Here's how the part is built. I have some questions about the finished solid (model axes, mm). A direction names the side the tool comes from. Coordinates: 2 decimals unless noted, no trailing zeros. Write each loop counter-clockwise with the first axis right and the second up, starting at its lowest first coordinate (ties: lowest second). Pieces come first, ordered by that corner, then holes.
Item 1: I want a section at A-A (y = -18.4). Please give me the cut outline in (x, z).
Item 2: For faces 1 (the face through (2.75, -8, -3)), 2 (the face through (4, -15, 4)), 3 (the face through (3, -7.8, 0)), 4 (the face through (5.25, -15, 0)), 5 (the face through (-3.25, 17, 0)), which set-ups out of +Z, -Z, +X, -X, +Y, -Y let a thin tool reach every point of the face, with its end or its side?
Item 3: If we mould it in two halves opening along Y, with no side actions, what happens to faces 6 (the face through (3, -19, -2.75)), 7 (the face through (4, -15, -4)), 8 (the face through (0, 25, 4)), 9 (the face through (4.757, -15.822, 0.338))? For each: pulls with the +Y half, pulls with the -Y half, needs draft (parallel to the pull), parting line crosses it, or undercut.
Item 4: I want a section at D-D (y = -24). Please give me the cut outline in (x, z).
Item 5: Please list where these lines run through material, in increasing order: line 1 (Y direction, x = -7, z = -4.25); line 2 (Y direction, x = 4.9, z = 0); line 3 (Y direction, x = 0.5, z = 0.25).
Item 6: I'm going to push flat-ended pins straight in: P1, Ø1.5, axis at y = 10.5, z = 2, coming from the -X side; P2, Ø4, axis at x = -6, z = 0.5, coming from the +Y side; P3, Ø0.8, axis at x = 4.5, y = -12.5, coming from the -Z side; P4, Ø4, axis at y = -14.5, z = -6.5, coming from the +X side. Where does each tip first touch, or does it pass through?
Item 7: I want a section at B-B (z = 0). Please give me the cut outline in (x, y), and give its area (3 significant figures).
Item 8: I want a section at C-C (x = 0). Please give me the cut outline in (y, z), and give its area (3 significant figures).
from build123d import *

# Parameters (mm, degrees)
SKETCH3_R           = 10
BOSS_EXTRUDE1_DEPTH = 25
SKETCH4_W           = 2.5
SKETCH4_H           = 8
BOSS_EXTRUDE2_DEPTH = 30
CUT_EXTRUDE1_REACH  = 37.108
SKETCH5_R           = 2.6
SKETCH6_W           = 5.5
SKETCH6_H           = 21.2
CUT_EXTRUDE2_DEPTH  = 1.5
SKETCH7_W           = 17
SKETCH7_H           = 7
CUT_EXTRUDE3_DEPTH  = 6
SKETCH8_W           = 2
SKETCH8_H           = 7
CUT_EXTRUDE4_DEPTH  = 4


with BuildPart() as part:
    # Sketch3 → Boss-Extrude1 (new body)
    with BuildSketch(Plane(origin=(0, 0, 0), x_dir=(1, 0, 0), z_dir=(0, 1, 0))):
        with Locations(Location((0, 0, 0), (0, 0, 270))):
            Circle(SKETCH3_R)
    extrude(amount=BOSS_EXTRUDE1_DEPTH)

    # Sketch4 → Boss-Extrude2 (add)
    with BuildSketch(Plane(origin=(0, 0, 0), x_dir=(-1, 0, 0), z_dir=(0, -1, 0))):
        with Locations((-4, 0)):
            Rectangle(SKETCH4_W, SKETCH4_H)
    extrude(amount=BOSS_EXTRUDE2_DEPTH)

    # Sketch5 → Cut-Extrude1 (cut, up to next)
    with BuildSketch(Plane(origin=(5.25, 0, 0), x_dir=(0, 0, -1), z_dir=(1, 0, 0)), mode=Mode.PRIVATE) as cut_extrude1_sk1:
        with Locations((0, -18.4)):
            Circle(SKETCH5_R)
    cut_extrude1_tool1 = extrude(cut_extrude1_sk1.sketch, amount=-CUT_EXTRUDE1_REACH, mode=Mode.PRIVATE) & part.part
    add(cut_extrude1_tool1.solids().sort_by_distance((5.25, -18.4, 0))[0], mode=Mode.SUBTRACT)

    # Sketch6 → Cut-Extrude2 (cut)
    with BuildSketch(Plane.ZY.offset(-2.75)):
        with Locations((0, -18.4)):
            Rectangle(SKETCH6_W, SKETCH6_H)
    extrude(amount=-CUT_EXTRUDE2_DEPTH, mode=Mode.SUBTRACT)

    # Sketch7 → Cut-Extrude3 (cut)
    with BuildSketch(Plane(origin=(0, 25, 0), x_dir=(1, 0, 0), z_dir=(0, 1, 0))):
        Rectangle(SKETCH7_W, SKETCH7_H)
    extrude(amount=-CUT_EXTRUDE3_DEPTH, mode=Mode.SUBTRACT)

    # Sketch8 → Cut-Extrude4 (cut)
    with BuildSketch(Plane(origin=(0, 19, 0), x_dir=(1, 0, 0), z_dir=(0, 1, 0))):
        with Locations((-2.25, 0)):
            Rectangle(SKETCH8_W, SKETCH8_H)
    extrude(amount=-CUT_EXTRUDE4_DEPTH, mode=Mode.SUBTRACT)


solid = part.part
Answer:
1. outline: (2.75, -4) - (5.25, -4) - (5.25, -2.6) - (4.25, -2.6) - (4.25, -2.75) - (2.75, -2.75) - close; (2.75, 2.75) - (4.25, 2.75) - (4.25, 2.6) - (5.25, 2.6) - (5.25, 4) - (2.75, 4) - close
2. face 1: +Z, -Z, -X, -Y
2. face 2: +Z, +X, -X, -Y
2. face 3: -X
2. face 4: +Z, -Z, +X, -Y
2. face 5: +Y
3. face 6: undercut
3. face 7: needs draft
3. face 8: pulls with the +Y half
3. face 9: undercut
4. outline: (2.75, -4) - (5.25, -4) - (5.25, 4) - (2.75, 4) - (2.75, 2.75) - (4.25, 2.75) - (4.25, -2.75) - (2.75, -2.75) - close
5. line 1: y = 0 to 25
5. line 2: y = -30 to -21, -15.8 to 19
5. line 3: y = 0 to 19
6. P1: stops at x = -9.92
6. P2: stops at y = 19
6. P3: stops at z = -4
6. P4: passes through
7. outline: (-10, 0) - (2.75, 0) - (2.75, -7.8) - (4.25, -7.8) - (4.25, -15.8) - (5.25, -15.8) - (5.25, 0) - (10, 0) - (10, 25) - (8.5, 25) - (8.5, 19) - (-1.25, 19) - (-1.25, 15) - (-3.25, 15) - (-3.25, 19) - (-8.5, 19) - (-8.5, 25) - (-10, 25) - close; (2.75, -30) - (5.25, -30) - (5.25, -21) - (4.25, -21) - (4.25, -29) - (2.75, -29) - close
7. area: 428 mm2
8. outline: (0, -10) - (25, -10) - (25, -3.5) - (19, -3.5) - (19, 3.5) - (25, 3.5) - (25, 10) - (0, 10) - close
8. area: 458 mm2
